Autodesk Inventor part; units mm, degrees
ref_plane "Start plane" through (0, 0, -20) normal (0, 0, 1) x (1, 0, 0)
ref_plane "End plane" through (0, 0, 770) normal (0, 0, 1) x (1, 0, 0)
ref_plane "Work Plane4" through (0, 20, 770) normal (0, -0.7071, 0.7071) x (1, 0, 0)
ref_plane "Start plane" through (0, 0, -20) normal (0, 0, 1) x (1, 0, 0)
ref_plane "End plane" through (0, 0, 770) normal (0, 0, 1) x (1, 0, 0)
sketch "Sketch" plane through (0, 0, 0) normal (0, 0, 1) x (1, 0, 0)
  line L0 (-20, -12) -> (-20, 12)
  line L1 (-12, 20) -> (12, 20)
  line L2 (20, 12) -> (20, -12)
  line L3 (12, -20) -> (-12, -20)
  arc A0 (-20, -12) -> (-12, -20) centre (-12, -12) ccw
  arc A1 (-12, 20) -> (-20, 12) centre (-12, 12) ccw
  arc A2 (20, 12) -> (12, 20) centre (12, 12) ccw
  arc A3 (12, -20) -> (20, -12) centre (12, -12) ccw
  arc A4 (-12, 16) -> (-16, 12) centre (-12, 12) ccw
  line L4 (-12, 16) -> (12, 16)
  arc A5 (16, 12) -> (12, 16) centre (12, 12) ccw
  line L5 (16, 12) -> (16, -12)
  arc A6 (12, -16) -> (16, -12) centre (12, -12) ccw
  line L6 (12, -16) -> (-12, -16)
  arc A7 (-16, -12) -> (-12, -16) centre (-12, -12) ccw
  line L7 (-16, -12) -> (-16, 12)
  line L8 (0, 30.3196) -> (0, -30.3196) construction
  line L9 (-30.3196, 0) -> (30.3196, 0) construction
  dimension "d7" = 8
  dimension "d10" = 40
  dimension "d11" = 40
  dimension "d12" = 4
  dimension "d15" = 20
  dimension "d16" = 20
extrude "Body" add sketch "Sketch" along normal up to surface (790 mm away) from surface at -20
sketch "Sketch3" plane through (0, 0, 0) normal (0, 0, 1) x (1, 0, 0)
  line L0 (0, 0) -> (10, 0)
ref_plane "Work Plane3" through (0, 0, 0) normal (0, -1, 0) x (1, 0, 0)
sketch "Sketch4" plane through (0, 0, 0) normal (0, -1, 0) x (1, 0, 0)
  line L0 (-2, -20) -> (12, -20)
  line L1 (-2, 770) -> (12, 770)
  dimension "d18" = 790
ref_plane "Work Plane4" through (0, 20, 770) normal (0, -0.7071, 0.7071) x (1, 0, 0)
split "Split1" plane through (0, 20, 770) removes the side toward (0, -0.7071, 0.7071)
ref_plane "Work Plane5" through (0, 20, -20) normal (0, -0.7071, -0.7071) x (1, 0, 0)
split "Split2" plane through (0, 20, -20) removes the side toward (0, -0.7071, -0.7071)
equation "\"d7\" = G_IR"
equation "\"d10\" = G_H"
equation "\"d11\" = G_W"
equation "\"d12\" = G_T"
equation "\"d15\" = 0.5 * d10"
equation "\"d16\" = 0.5 * d11"
equation "\"d3\" = G_L"
equation "\"G_W\" = 40"
equation "\"G_H\" = 40"
equation "\"G_T\" = 4"
equation "\"G_IR\" = 8"
equation "\"G_L\" = d18"
equation "\"G_OFFSET_START\" = 20"
equation "\"G_OFFSET_END\" = 20"
equation "\"d13\" = -G_OFFSET_START"
equation "\"B_L\" = 750"
properties part number "DIN EN 10219-2 - 40 x 40 x 4  - 790" material "Steel, Mild"
Geometry check sheet. Reference: the model listing, model coordinates, mm. A direction names the side the tool comes from. Round coordinates to 2 decimals unless told otherwise and drop trailing zeros. Loops run counter-clockwise (first coordinate to the right, second up) from the corner with the lowest first, then second, coordinate; pieces in that order, holes last. Notation, with made-up numbers: (28.5, 53.25) - (86.5, 53.25) arc R35 cw to (86.5, 87.25) - close; hole circle Ø5 at (67.5, 36.5). An arc over 180 degrees is marked (long way). Write each question's results on one line, items separated by ' | '. Start each with the question number.
Q1. Gauge pin test, flat ends, axial feed: P1, Ø1, axis at y = -15.5, z = 80.5, coming from the +X side; P2, Ø1, axis at y = 14, z = 320, coming from the -X side; P3, Ø4, axis at x = -4.5, y = 16, coming from the +Z side. Record the tip position at first contact, or that the pin passes through.
Q2. Cross-section at C-C on x = -3.5. Enter the section's corners in (y, z).
Q3. Release check for a two-part mould opening along Y. For faces 3 (the flat face through (-16.4, 0.1, -0.1)), 4 (the flat face through (20, 0, 370)), 5 (the flat face through (-16, 0, 370)) record: +Y half, -Y half, draft (parallel to the pull), parting line (faces both ways), or undercut.
Q4. Cross-section at A-A on z = 675.5. Enter the section's corners in (x, y).
Q5. Thickness scan on line 1 (Y direction, x = -3.5, z = 21.5); line 2 (X direction, y = 13.5, z = 176). Record the ranges inside material, lowest first. Write a range as [from, to].
Q6. Cross-section at B-B on y = -2.5. Enter the section's corners in (x, z).
Q7. Access from +Z, -Z, +X, -X, +Y, -Y to the whole of each face (thin tool, end or side, straight path). Record for faces 1 (the flat face through (-20, 0, 370)), 2 (the flat face through (16, 0, 370)).
Answers below:
1) P1: stops at x = 19.42 | P2: stops at x = -19.86 | P3: stops at z = 768
2) outline: (-20, 20) - (-16, 16) - (-16, 734) - (-20, 730) - close; (16, -16) - (20, -20) - (20, 770) - (16, 766) - close
3) face 3: -Y half | face 4: draft | face 5: undercut
4) outline: (-20, -12) arc R8 ccw to (-12, -20) - (12, -20) arc R8 ccw to (20, -12) - (20, 12) arc R8 ccw to (12, 20) - (-12, 20) arc R8 ccw to (-20, 12) - close; hole (-16, -12) arc R4 ccw to (-12, -16) - (12, -16) arc R4 ccw to (16, -12) - (16, 12) arc R4 ccw to (12, 16) - (-12, 16) arc R4 ccw to (-16, 12) - close
5) line 1: y = [-20, -16], [16, 20] | line 2: x = [-19.86, -15.71], [15.71, 19.86]
6) outline: (-20, 2.5) - (-16, 2.5) - (-16, 747.5) - (-20, 747.5) - close; (16, 2.5) - (20, 2.5) - (20, 747.5) - (16, 747.5) - close
7) face 1: +Z, -Z, -X, +Y, -Y | face 2: +Z, -Z
